Geometry: final body of the model. Coordinates: model frame, mm. Face numbers are marked on the shaded views. Coordinates: 2 decimals unless noted, no trailing zeros. Loops run counter-clockwise (first coordinate to the right, second up) from the corner with the lowest first, then second, coordinate; pieces in that order, holes last. Notation, with made-up numbers: (83.5, 1.5) -> (109.5, 1.5) arc R6 ccw to (109.5, 8.5) -> close; hole circle Ø10 at (-25.5, 63.25). An arc over 180 degrees is marked (long way). One line per item, written item: value. Start each with the question number.
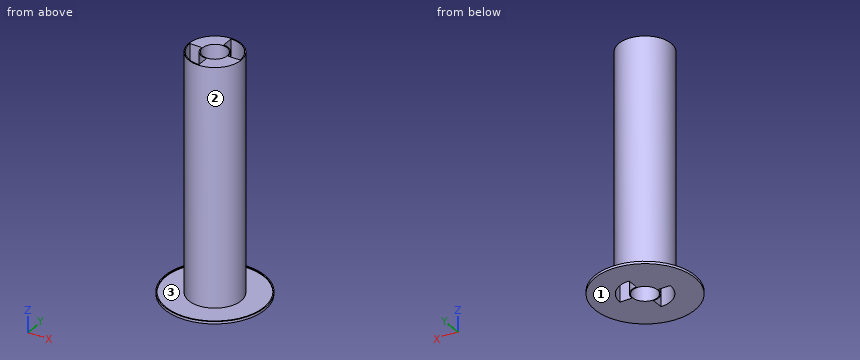
from build123d import *

# Parameters (mm, degrees)
F0_R     = 105
F0_R_2   = 55
F0_R_3   = 26
F1_DEPTH = 3
F2_DEPTH = 500
F3_DEPTH = 500
F4_R     = 105
F4_R_2   = 103
F5_DEPTH = 2
F6_DEPTH = 500
F7_DEPTH = 25


# Not quite as in the source:
# - after a boolean that leaves OpenCascade's solid faulty, fix() repairs it


with BuildPart() as f1:
    # F0 (on Top) → F1 (new body)
    with BuildSketch(Plane.XY):
        Circle(F0_R)
        Circle(F0_R_2, mode=Mode.SUBTRACT)
        Circle(F0_R_2)
        with BuildLine():
            ThreePointArc((0, 53), (37.4766594029, 37.4766594029), (53, 0))
            ThreePointArc((53, 0), (37.4766594029, -37.4766594029), (0, -53))
            ThreePointArc((0, -53), (-37.4766594029, -37.4766594029), (-53, 0))
            ThreePointArc((-53, 0), (-37.4766594029, 37.4766594029), (0, 53))
        make_face(mode=Mode.SUBTRACT)
        with BuildLine():
            ThreePointArc((0, 28), (19.7989898732, 19.7989898732), (28, 0))
            Line((28, 0), (53, 0))
            ThreePointArc((53, 0), (37.4766594029, 37.4766594029), (0, 53))
            Line((0, 53), (0, 28))
        make_face()
        with BuildLine():
            ThreePointArc((-28, 0), (-19.7989898732, 19.7989898732), (0, 28))
            Line((0, 28), (0, 53))
            ThreePointArc((0, 53), (-37.4766594029, 37.4766594029), (-53, 0))
            Line((-53, 0), (-28, 0))
        make_face()
        with BuildLine():
            Line((0, -53), (0, -28))
            ThreePointArc((0, -28), (-19.7989898732, -19.7989898732), (-28, 0))
            Line((-28, 0), (-53, 0))
            ThreePointArc((-53, 0), (-37.4766594029, -37.4766594029), (0, -53))
        make_face()
        with BuildLine():
            Line((53, 0), (28, 0))
            ThreePointArc((28, 0), (19.7989898732, -19.7989898732), (0, -28))
            Line((0, -28), (0, -53))
            ThreePointArc((0, -53), (37.4766594029, -37.4766594029), (53, 0))
        make_face()
        with BuildLine():
            ThreePointArc((0, -28), (19.7989898732, -19.7989898732), (28, 0))
            ThreePointArc((28, 0), (19.7989898732, 19.7989898732), (0, 28))
            ThreePointArc((0, 28), (-19.7989898732, 19.7989898732), (-28, 0))
            ThreePointArc((-28, 0), (-19.7989898732, -19.7989898732), (0, -28))
        make_face()
        Circle(F0_R_3, mode=Mode.SUBTRACT)
    extrude(amount=F1_DEPTH)

    # F0 (on Top) → F2 (join)
    with BuildSketch(Plane.XY):
        with BuildLine():
            ThreePointArc((0, -28), (19.7989898732, -19.7989898732), (28, 0))
            ThreePointArc((28, 0), (19.7989898732, 19.7989898732), (0, 28))
            ThreePointArc((0, 28), (-19.7989898732, 19.7989898732), (-28, 0))
            ThreePointArc((-28, 0), (-19.7989898732, -19.7989898732), (0, -28))
        make_face()
        Circle(F0_R_3, mode=Mode.SUBTRACT)
    extrude(amount=F2_DEPTH)

    # F0 (on Top) → F3 (join)
    with BuildSketch(Plane.XY):
        Circle(F0_R_2)
        with BuildLine():
            ThreePointArc((0, 53), (37.4766594029, 37.4766594029), (53, 0))
            ThreePointArc((53, 0), (37.4766594029, -37.4766594029), (0, -53))
            ThreePointArc((0, -53), (-37.4766594029, -37.4766594029), (-53, 0))
            ThreePointArc((-53, 0), (-37.4766594029, 37.4766594029), (0, 53))
        make_face(mode=Mode.SUBTRACT)
    extrude(amount=F3_DEPTH)

    # F4 (on face) → F5 (join)
    with BuildSketch(Plane.XY.offset(3)):
        Circle(F4_R)
        Circle(F4_R_2, mode=Mode.SUBTRACT)
    extrude(amount=F5_DEPTH)

    # F0 (on Top) → F6 (join)
    with BuildSketch(Plane.XY):
        with BuildLine():
            ThreePointArc((-28, 0), (-19.7989898732, 19.7989898732), (0, 28))
            Line((0, 28), (0, 53))
            ThreePointArc((0, 53), (-37.4766594029, 37.4766594029), (-53, 0))
            Line((-53, 0), (-28, 0))
        make_face()
        with BuildLine():
            Line((53, 0), (28, 0))
            ThreePointArc((28, 0), (19.7989898732, -19.7989898732), (0, -28))
            Line((0, -28), (0, -53))
            ThreePointArc((0, -53), (37.4766594029, -37.4766594029), (53, 0))
        make_face()
    extrude(amount=F6_DEPTH)

    # F0 (on Top) → F7 (cut)
    with BuildSketch(Plane.XY):
        with BuildLine():
            Line((0, -53), (0, -28))
            ThreePointArc((0, -28), (-19.7989898732, -19.7989898732), (-28, 0))
            Line((-28, 0), (-53, 0))
            ThreePointArc((-53, 0), (-37.4766594029, -37.4766594029), (0, -53))
        make_face()
        with BuildLine():
            ThreePointArc((0, 28), (19.7989898732, 19.7989898732), (28, 0))
            Line((28, 0), (53, 0))
            ThreePointArc((53, 0), (37.4766594029, 37.4766594029), (0, 53))
            Line((0, 53), (0, 28))
        make_face()
    extrude(amount=F7_DEPTH, mode=Mode.SUBTRACT)

    add(f1.part.fix(), mode=Mode.REPLACE)


solid = f1.part
1. Section C-C on x = 36. Return the cut outline in (y, z).
2. Section D-D on x = -64. Return the cut outline in (y, z).
3. Pin query (flat end, axial travel): pin 1 Ø1.5 at (x, y) = (-77.5, -1) entering from +Z; pin 2 Ø8 at (y, z) = (-38.5, 169) entering from -X; pin 3 Ø2 at (y, z) = (-8.5, 224.5) entering from -X. Return the tip coordinate at first contact, or that it passes through.
4. Section B-B on y = -6. Return the cut outline in (x, z), plus the area to 3 significant figures.
5. Draft query along X for the marked faces 1, 2 and 3. Return one class per face: released by +X, released by -X, zero draft, split by the parting line, or undercut.
6. Line query: L1, parallel to Y at x = -15, z = 38; L2, parallel to Y at x = 11, z = 398; L3, parallel to Z at x = 45.5, y = 85.5. Output: solid intervals per line, ascending. Write a range as [from, to].
7. Section A-A on z = 161.5. Return the cut outline in (x, y).
Checks:
1. outline: (-98.64, 0) -> (0, 0) -> (0, 500) -> (-41.58, 500) -> (-41.58, 3) -> (-96.5, 3) -> (-96.5, 5) -> (-98.64, 5) -> close; (38.9, 0) -> (98.64, 0) -> (98.64, 5) -> (96.5, 5) -> (96.5, 3) -> (41.58, 3) -> (41.58, 500) -> (38.9, 500) -> close
2. outline: (-83.24, 0) -> (83.24, 0) -> (83.24, 5) -> (80.7, 5) -> (80.7, 3) -> (-80.7, 3) -> (-80.7, 5) -> (-83.24, 5) -> close
3. pin 1: z = 3
3. pin 2: x = -42.83
3. pin 3: x = -54.49
4. outline: (-104.83, 0) -> (-52.66, 0) -> (-52.66, 500) -> (-54.67, 500) -> (-54.67, 3) -> (-102.83, 3) -> (-102.83, 5) -> (-104.83, 5) -> close; (-27.35, 0) -> (-25.3, 0) -> (-25.3, 500) -> (-27.35, 500) -> close; (25.3, 0) -> (104.83, 0) -> (104.83, 5) -> (102.83, 5) -> (102.83, 3) -> (54.67, 3) -> (54.67, 500) -> (25.3, 500) -> close
4. area: 17,000 mm²
5. face 1: zero draft
5. face 2: split by the parting line
5. face 3: undercut
6. L1: [-52.92, -50.83], [-23.64, -21.24], [21.24, 52.92]
6. L2: [-53.89, -23.56], [23.56, 25.75], [51.85, 53.89]
6. L3: [0, 3]
7. outline: circle Ø110 at (0, 0); hole (-53, 0) arc R53 ccw to (0, -53) -> (0, -28) arc R28 cw to (-28, 0) -> close; hole circle Ø52 at (0, 0); hole (0, 28) arc R28 cw to (28, 0) -> (53, 0) arc R53 ccw to (0, 53) -> close
